Part model, mm, in its own coordinate system. Round coordinates to 2 decimals unless told otherwise and drop trailing zeros. Loops run counter-clockwise (first coordinate to the right, second up) from the corner with the lowest first, then second, coordinate; pieces in that order, holes last. Notation, with made-up numbers: M -10.5,6 L 45.5,6 A27 ccw 45.5,30 Z; hole C 57.5,-28 d10. An arc over 180 degrees is marked long. Answer as CSV lines item,"result". Start each with the question number.
Item 1: Wall check: line 1 (X direction, y = 209, z = -2.5); line 2 (X direction, y = 208.5, z = -1.8); line 3 (Y direction, x = -44, z = -0.45). Give the ranges that are in metal, low to high.
Item 2: Band-saw the part on B-B (y = 206). Give the cut face in (x, z) (3 decimals), and give its area (3 significant figures).
Item 3: Band-saw the part on A-A (y = 279.5). Give the cut face in (x, z) (3 decimals).
Item 4: Drop a flat-ended pin along its axis: pin 1 Ø1 at (y, z) = (65.5, -0.5) entering from +X. Give the stop position or say it passes through.
Autodesk Inventor part; units mm, degrees
ref_plane "YZ Plane" through (0, 0, 0) normal (1, 0, 0) x (0, 1, 0)
ref_plane "XZ Plane" through (0, 0, 0) normal (0, 1, 0) x (-1, 0, 0)
ref_plane "XY Plane" through (0, 0, 0) normal (0, 0, 1) x (1, 0, 0)
sketch "Sketch1" plane through (0, 0, 0) normal (0, 0, 1) x (1, 0, 0)
  line L0 (76.2, -12.7) -> (381, -12.7) construction
  line L1 (-76.2, -12.7) -> (-381, -12.7) construction
  line L2 (-76.2, 0) -> (-381, 0) construction
  line L3 (76.2, 0) -> (381, 0) construction
  line L4 (0, -116.2267) -> (0, 608.4603)
  line L5 (0, -12.7) -> (-122.0009, -12.7)
  line L6 (-122.0009, -12.7) -> (-122.0009, 0)
  line L7 (0, 394.3626) -> (-6.35, 394.3626)
  line L8 (-52.4512, 312.4765) -> (-60.2591, 93.2692)
  spline S0 degree 3 poles (-122.0009, 0) (-64.2705, 0) (-61.6839, 53.2691) (-60.2591, 93.2692) knots 0 0 0 0 1 1 1 1
  line L9 (-127.2981, 0) -> (-116.7037, 0) construction
  arc A0 (-126.2344, 0.0955) -> (-117.7675, 0.0955) centre (-122.0009, 93.8482) ccw construction
  line L10 (52.4512, 312.4765) -> (60.2591, 93.2692)
  line L11 (0, 394.3626) -> (6.35, 394.3626)
  spline S1 degree 3 poles (122.0009, 0) (64.2705, 0) (61.6839, 53.2691) (60.2591, 93.2692) knots 0 0 0 0 1 1 1 1
  line L12 (127.2981, 0) -> (116.7037, 0) construction
  arc A1 (117.7675, 0.0955) -> (126.2344, 0.0955) centre (122.0009, 93.8482) ccw construction
  line L13 (0, -12.7) -> (122.0009, -12.7)
  line L14 (122.0009, -12.7) -> (122.0009, 0)
  spline S2 degree 4 poles (-6.35, 394.3626) (-6.35, 370.6692) (-16.2148, 349.4175) (-49.2512, 345.2253) (-52.0931, 322.5296) (-52.4512, 312.4765) knots 0 0 0 0 0 0.529809 1 1 1 1 1
  line L15 (-6.35, 421.2444) -> (-6.35, 367.4808) construction
  arc A2 (-7.9378, 373.0956) -> (-7.9378, 415.6296) centre (-149.5647, 394.3626) ccw construction
  spline S3 degree 4 poles (6.35, 394.3626) (6.35, 349.6419) (36.5958, 353.9783) (51.6896, 333.8574) (52.4512, 312.4765) knots 0 0 0 0 0 1 1 1 1 1
  line L16 (6.35, 421.2444) -> (6.35, 367.4808) construction
  arc A3 (7.9378, 415.6296) -> (7.9378, 373.0956) centre (149.5647, 394.3626) ccw construction
  line L17 (-23.1287, 353.4652) -> (-48.6526, 335.307) construction
  arc A4 (-25.2872, 350.8986) -> (-45.5201, 336.5045) centre (17.5347, 269.2893) ccw construction
  point P0 (0, 0)
  point P1 (-35.8906, 344.3861)
  point P2 (35.8906, 344.3861)
  dimension "d0" = 6.35
extrude "Extrusion1" add sketch "Sketch1" against normal blind 3.175
properties part number "Plate" material "High Impact Polystyrene"
Answer block:
1,line 1,"x = -56.14 to 56.14"
1,line 2,"x = -56.15 to 56.15"
1,line 3,"y = -12.7 to 337.41"
2,outline,"M -56.244,-3.175 L 56.244,-3.175 L 56.244,0 L -56.244,0 Z"
2,area,"357 mm^2"
3,outline,"M -53.626,-3.175 L 53.626,-3.175 L 53.626,0 L -53.626,0 Z"
4,pin 1,"stops at x = 62.01"
